from build123d import *

# Parameters (mm, degrees)
F1_DEPTH = 63.5
F2_DEPTH = 7.9375
F3_DEPTH = 25.4
F5_R     = 6.35


with BuildPart() as f1:
    # F0 (on Front) → F1 (new body, symmetric)
    with BuildSketch(Plane.XZ):
        Polygon((-41.275, -9.525), (41.275, -9.525), (41.275, 9.525), (22.225, 9.525), (-41.275, 9.525), align=None)
    extrude(amount=F1_DEPTH, both=True)

    # F0 (on Front) → F2 (join, symmetric)
    with BuildSketch(Plane.XZ):
        with BuildLine():
            add(Edge.make_bspline(
                [(-41.275, 9.525), (-28.1295553006, 44.6239538406), (21.5320084104, 56.6569118674), (56.3533917414, 57.1409138543)],
                knots=[0, 0, 0, 0, 108.5115602051, 108.5115602051, 108.5115602051, 108.5115602051], degree=3))
            Line((-41.275, 9.525), (22.225, 9.525))
            Line((22.225, 9.525), (22.225, 22.225))
            ThreePointArc((22.225, 22.225), (32.1742400673, 46.6374361911), (56.3533917414, 57.1409138543))
        make_face()
    extrude(amount=F2_DEPTH, both=True)

    # F0 (on Front) → F3 (join, symmetric)
    with BuildSketch(Plane.XZ):
        with BuildLine():
            Line((22.225, 9.525), (41.275, 9.525))
            Line((41.275, 9.525), (41.275, 22.225))
            ThreePointArc((41.275, 22.225), (45.9246798487, 33.4503201513), (57.15, 38.1))
            Line((57.15, 38.1), (60.325, 38.1))
            Line((60.325, 38.1), (60.325, 57.15))
            Line((60.325, 57.15), (57.15, 57.15))
            add(Edge.make_bspline(
                [(56.3533917414, 57.1409138543), (56.6198041666, 57.1446168704), (56.8853479194, 57.1476438664), (57.15, 57.15)],
                knots=[108.5115602051, 108.5115602051, 108.5115602051, 108.5115602051, 109.3417635215, 109.3417635215, 109.3417635215, 109.3417635215], degree=3))
            ThreePointArc((56.3533917414, 57.1409138543), (32.1742400673, 46.6374361911), (22.225, 22.225))
            Line((22.225, 22.225), (22.225, 9.525))
        make_face()
        Polygon((60.325, 57.15), (60.325, 38.1), (80.6127000995, 38.1), (85.725, 38.1), (85.725, 57.15), (80.6127000995, 57.15), align=None)
    extrude(amount=F3_DEPTH, both=True)

    # F0 (on Front) → F4 (revolve)
    with BuildSketch(Plane.XZ):
        Polygon((85.725, 57.15), (85.725, 38.1), (111.125, 38.1), (111.125, 66.675), (85.725, 66.675), align=None)
    revolve(axis=Axis((85.725, 0, 52.3875), (0, 0, -1)))

    # F5
    f5_edges = [f1.edges().sort_by_distance(p)[0] for p in [
        (41.275, -63.5, 0),
        (-41.275, -63.5, 0),
        (-41.275, 63.5, 0),
        (41.275, 63.5, 0),
    ]]
    fillet(f5_edges, radius=F5_R)


solid = f1.part
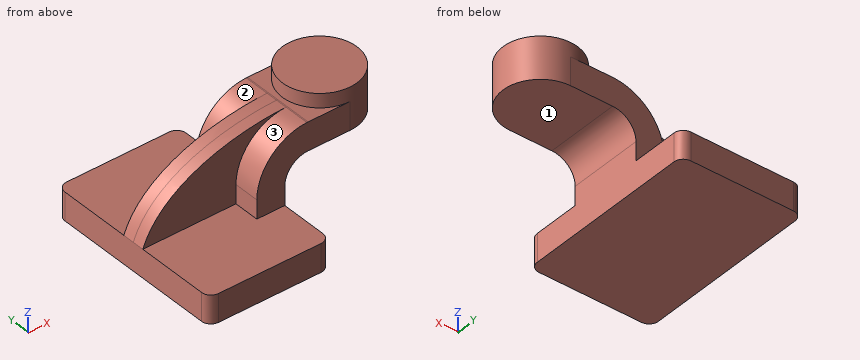
Could you check a few things on this model? Use its own coordinates, in mm. Face numbers are marked on the shaded views. A direction names the side the tool comes from. Give positions to 0.01 mm unless a question says otherwise; leave off trailing zeros. Order: outer loops, then holes, each group sorted by start corner. A loop starts at its lowest first (then second) coordinate and runs counter-clockwise, first axis right, second up.
1. Which directions (+Z, -Z, +X, -X, +Y, -Y) give clear straight access to the entire face, cutting with the end or side of a thin tool? Please do the marked faces 1, 2 and 3.
Answers below:
face 1: -Z, +X, +Y, -Y
face 2: +Z, -X, +Y
face 3: +Z, -X, -Y
2. For pin 1 (1 mm diameter, centred on y = 12, z = 12, fed in from -X) (3 decimals); pin 2 (8 mm diameter, centred on y = -14.5, z = 33.5, fed in from -X); pin 3 (24 mm diameter, centred on x = 64, z = 35.5, fed in from +Y); pin 4 (14 mm diameter, centred on y = -20.5, z = 14, fed in from -X) (3 decimals), each with a flat end and sliding along its axis, tell me the tip position at first contact or that it passes through.
Answers below:
pin 1: stops at x = 22.225
pin 2: stops at x = 22.99
pin 3: stops at y = 25.4
pin 4: stops at x = -41.275
3. I need wall thicknesses on L1, parallel to Z at x = 18, y = 14.5 (3 decimals); L2, parallel to Z at x = 70, y = -22.5; L3, parallel to Y at x = 35, z = 39.5. Which ranges of each line are inside material? Lowest first, please.
Answers below:
L1: z = -9.525 to 9.525
L2: z = 38.1 to 57.15
L3: y = -25.4 to 25.4
4. Suppose I cut it at B-B (x = 74). Write out the boundary of the cut face in (y, z) (3 decimals).
Answers below:
outline: (-25.4, 38.1) - (25.4, 38.1) - (25.4, 57.15) - (22.532, 57.15) - (22.532, 66.675) - (-22.532, 66.675) - (-22.532, 57.15) - (-25.4, 57.15) - close
5. Suppose I cut it at A-A (z = 4.5). Write out the boundary of the cut face in (x, y) (3 decimals).
Answers below:
outline: (-41.275, -57.15) arc R6.35 ccw to (-34.925, -63.5) - (34.925, -63.5) arc R6.35 ccw to (41.275, -57.15) - (41.275, 57.15) arc R6.35 ccw to (34.925, 63.5) - (-34.925, 63.5) arc R6.35 ccw to (-41.275, 57.15) - close
6. Suppose I cut it at C-C (x = 91). Write out the boundary of the cut face in (y, z) (3 decimals), plus the area to 3 significant figures.
Answers below:
outline: (-24.846, 38.1) - (24.846, 38.1) - (24.846, 66.675) - (-24.846, 66.675) - close
area: 1,420 mm2
